Input: part model. Units: mm. Frame: model coordinates. Coordinates: 2 decimals unless noted, no trailing zeros. Write each loop counter-clockwise with the first axis right and the second up, starting at its lowest first coordinate (ties: lowest second). Pieces come first, ordered by that corner, then holes. Notation, with made-up numbers: (-27.75, -35.75) - (10.25, -35.75) arc R26 ccw to (10.25, -18.75) - close; hole circle Ø2 at (-30.5, 65). An arc over 180 degrees is marked (long way). One line per question, with ' | ' between items. Start each with the question number.
1) Section query C-C on x = -17.34. Return loops of the section in (y, z), and give its area (3 significant figures).
2) Section query A-A on z = 6.25. Return loops of the section in (x, y) (1 decimal), and give its area (3 significant figures).
3) Line query: line 1 (X direction, y = -8, z = 5); line 2 (Y direction, x = -13, z = 15); line 3 (X direction, y = 9.5, z = 3.75). Output: solid intervals per line, ascending.
4) Draft query along X for faces 1 (the cylindrical face through (-1.924, -5.359, 7.888)), 2 (the cylindrical face through (-9.56, 15.912, 7.888)), 3 (the cylindrical face through (-22.48, -6.97, 7.89)), 4 (the cylindrical face through (-11.91, -10.46, 7.89)). Return one class per face: released by +X, released by -X, zero draft, split by the parting line, or undercut.
5) Section query B-B on y = 13.5. Return loops of the section in (x, z), and give its area (3 significant figures).
6) First-contact query: P1, Ø5, axis at x = -23, z = 5.5, coming from the -Y side; P2, Ø1, axis at x = -19, z = 12, coming from the -Y side; P3, Ø4, axis at x = -3, z = 12.5, coming from the -Y side. Flat tips, straight axial feed; report the tip coordinate or a pass-through.
```python
from build123d import *

# Parameters (mm, degrees)
CYLINDER_R        = 1.5
CYLINDER_DEPTH    = 18
ARRAY_COUNT       = 8
CYLINDER001_R     = 14.5
CYLINDER001_DEPTH = 16


with BuildPart() as array:
    # Cylinder → Cylinder (new body)
    with BuildSketch(Plane.XY):
        Circle(CYLINDER_R)
    extrude(amount=CYLINDER_DEPTH)

    # Array: Array ×8 about axis
    array_axis = Axis((-13.22, 4.12, 0), (0, 0, 1))


with BuildPart() as array_1:
    add(array.part)
    for i in range(1, ARRAY_COUNT):
        add(array.part.rotate(array_axis, i * 360 / ARRAY_COUNT))


with BuildPart() as cut:
    # Cylinder001 → Cylinder001 (new body)
    with BuildSketch(Plane(origin=(-13, 4, 0), x_dir=(1, 0, 0), z_dir=(0, 0, 1))):
        Circle(CYLINDER001_R)
    extrude(amount=CYLINDER001_DEPTH)

    # Cut: cut Array
    add(array_1.part, mode=Mode.SUBTRACT)


solid = cut.part
```
Answer key:
1) outline: (-7.6, 0) - (17.84, 0) - (17.84, 16) - (-7.6, 16) - close | area: 407 mm²
2) outline: (-27.2, 6.9) arc R14.5 ccw to (-26.5, -1.2) arc R1.5 cw (long way) to (-25.2, -3.8) arc R14.5 ccw to (-18.8, -9.3) arc R1.5 cw (long way) to (-16.3, -10.1) arc R14.5 ccw to (-7.5, -9.4) arc R1.5 cw (long way) to (-5.3, -8.3) arc R14.5 ccw to (0.4, -1.4) arc R1.5 cw (long way) to (1.2, 0.9) arc R14.5 ccw to (0.3, 9.8) arc R1.5 cw (long way) to (-0.9, 12.1) arc R14.5 ccw to (-7.6, 17.5) arc R1.5 cw (long way) to (-10.3, 18.2) arc R14.5 ccw to (-18.5, 17.4) arc R1.5 cw (long way) to (-21.1, 16) arc R14.5 ccw to (-26.3, 9.7) arc R1.5 cw (long way) to start | area: 618 mm²
3) line 1: -21.14 to -18.36, -16.32 to -8.28, -5.29 to -4.86 | line 2: -10.5 to 18.5 | line 3: -25.63 to -2.03, 0.11 to 0.42
4) face 1: released by +X | face 2: undercut | face 3: released by -X | face 4: split by the parting line
5) outline: (-23.95, 0) - (-2.05, 0) - (-2.05, 16) - (-23.95, 16) - close | area: 351 mm²
6) P1: y = -8.41 | P2: y = -9.28 | P3: y = -8.09
